Build history of the part. All positions in model axes, mm. A direction names the side the tool comes from. Give positions to 0.01 mm unless a question says otherwise; leave off trailing zeros. Loops run counter-clockwise (first coordinate to the right, second up) from the corner with the lowest first, then second, coordinate; pieces in that order, holes last. Notation, with made-up numbers: (26, 65) -> (78, 65) arc R16 cw to (78, 71) -> close; hole circle Ø3 at (26, 50.25). An arc over 180 degrees is marked (long way). Answer as a JSON object with one key per item and string values. Group by question number.
from build123d import *

# Parameters (mm, degrees)
F0_W         = 39
F0_H         = 55.5
F0_W_2       = 35
F0_H_2       = 51.5
F1_DEPTH     = 37
F3_DEPTH     = 56
F4_DEPTH     = 2
F5_R         = 2.5
F6_DEPTH     = 3
F7_W         = 6
F7_H         = 2
F8_DEPTH     = 40
F9_T1_DEPTH  = 47.5
F9_T3_DEPTH  = 31
F9_T5_DEPTH  = 43
F9_S9_W      = 4
F9_S9_H      = 4
F9_T10_DEPTH = 4
F9_S15_W     = 4
F9_S15_H     = 4
F9_T16_DEPTH = 4
F9_S21_W     = 4
F9_S21_H     = 4
F9_T22_DEPTH = 4
F9_S27_W     = 4
F9_S27_H     = 4
F9_T28_DEPTH = 4


# Not quite as in the source:
# - a fillet or chamfer that OpenCascade refuses, or shapes differently, is made with other operations: its cross-section is extruded or revolved along the edge and cut away or added


with BuildPart() as f1:
    # F0 (on Top) → F1 (new body)
    with BuildSketch(Plane.XY):
        Rectangle(F0_W, F0_H)
        Rectangle(F0_W_2, F0_H_2, mode=Mode.SUBTRACT)
    extrude(amount=F1_DEPTH)

    # F2 (on face) → F3 (cut)
    with BuildSketch(Plane(origin=(0, 27.75, 0), x_dir=(-1, 0, 0), z_dir=(0, 1, 0))):
        with BuildLine():
            Line((19.5, 37), (-19.5, 37))
            ThreePointArc((-19.5, 37), (0, 27.8760560333), (19.5, 37))
        make_face()
    extrude(amount=-F3_DEPTH, mode=Mode.SUBTRACT)

    # F0 (on Top) → F4 (join)
    with BuildSketch(Plane.XY):
        Rectangle(F0_W_2, F0_H_2)
    extrude(amount=F4_DEPTH)

    # F5 (on face) → F6 (cut)
    with BuildSketch(Plane(origin=(0, 27.75, 0), x_dir=(-1, 0, 0), z_dir=(0, 1, 0))):
        with Locations((0, 4.8760560333)):
            Circle(F5_R)
    extrude(amount=-F6_DEPTH, mode=Mode.SUBTRACT)

    # F7 (on face) → F8 (cut)
    with BuildSketch(Plane(origin=(-19.5, 0, 0), x_dir=(0, -1, 0), z_dir=(-1, 0, 0))):
        with Locations((-19.75, 31.5)):
            Rectangle(F7_W, F7_H)
        with Locations((-6.75, 31.5)):
            Rectangle(F7_W, F7_H)
        with Locations((6.25, 31.5)):
            Rectangle(F7_W, F7_H)
        with Locations((19.25, 31.5)):
            Rectangle(F7_W, F7_H)
    extrude(amount=-F8_DEPTH, mode=Mode.SUBTRACT)

    # F9: fillet of radius 4 on 8 edges, made by hand

    # F9_s2 → F9_t1 (cut)
    with BuildSketch(Plane.XZ.offset(-23.75)):
        with BuildLine():
            ThreePointArc((-15.5, 0), (-18.3284271247, 1.1715728753), (-19.5, 4))
            Line((-19.5, 4), (-19.5, 0))
            Line((-19.5, 0), (-15.5, 0))
        make_face()
        with BuildLine():
            ThreePointArc((19.5, 4), (18.3284271247, 1.1715728753), (15.5, 0))
            Line((15.5, 0), (19.5, 0))
            Line((19.5, 0), (19.5, 4))
        make_face()
    extrude(amount=F9_T1_DEPTH, mode=Mode.SUBTRACT)

    # F9_s4 → F9_t3 (cut)
    with BuildSketch(Plane.YZ.offset(-15.5)):
        with BuildLine():
            ThreePointArc((23.75, 0), (26.5784271247, 1.1715728753), (27.75, 4))
            Line((27.75, 4), (27.75, 0))
            Line((27.75, 0), (23.75, 0))
        make_face()
        with BuildLine():
            ThreePointArc((-27.75, 4), (-26.5784271247, 1.1715728753), (-23.75, 0))
            Line((-23.75, 0), (-27.75, 0))
            Line((-27.75, 0), (-27.75, 4))
        make_face()
    extrude(amount=F9_T3_DEPTH, mode=Mode.SUBTRACT)

    # F9_s6 → F9_t5 (cut)
    with BuildSketch(Plane.XY.offset(4)):
        with BuildLine():
            ThreePointArc((-15.5, -27.75), (-18.3284271247, -26.5784271247), (-19.5, -23.75))
            Line((-19.5, -23.75), (-19.5, -27.75))
            Line((-19.5, -27.75), (-15.5, -27.75))
        make_face()
        with BuildLine():
            ThreePointArc((19.5, -23.75), (18.3284271247, -26.5784271247), (15.5, -27.75))
            Line((15.5, -27.75), (19.5, -27.75))
            Line((19.5, -27.75), (19.5, -23.75))
        make_face()
        with BuildLine():
            ThreePointArc((19.5, 23.75), (18.3284271247, 26.5784271247), (15.5, 27.75))
            Line((15.5, 27.75), (19.5, 27.75))
            Line((19.5, 27.75), (19.5, 23.75))
        make_face()
        with BuildLine():
            ThreePointArc((-15.5, 27.75), (-18.3284271247, 26.5784271247), (-19.5, 23.75))
            Line((-19.5, 23.75), (-19.5, 27.75))
            Line((-19.5, 27.75), (-15.5, 27.75))
        make_face()
    extrude(amount=F9_T5_DEPTH, mode=Mode.SUBTRACT)


with BuildPart() as f9_tool8:
    # F9_s9 → F9_t10 (new body)
    with BuildSketch(Plane.XY.offset(4)):
        with Locations((-17.5, 25.75)):
            Rectangle(F9_S9_W, F9_S9_H)
    extrude(amount=-F9_T10_DEPTH)

    # F9_s11 → F9_t12 (revolve, cut)
    with BuildSketch(Plane(origin=(-15.5, 23.75, 4), x_dir=(0.7071067812, -0.7071067812, 0), z_dir=(0.7071067812, 0.7071067812, 0))):
        with BuildLine():
            ThreePointArc((0, -4), (4, 0), (0, 4))
            Line((0, 4), (0, -4))
        make_face()
    revolve(axis=Axis((-15.5, 23.75, 4), (0, 0, -1)), mode=Mode.SUBTRACT)


with BuildPart() as f1_1:
    add(f1.part)

    # F9_t7: cut F9_tool8
    add(f9_tool8.part, mode=Mode.SUBTRACT)


with BuildPart() as f9_tool14:
    # F9_s15 → F9_t16 (new body)
    with BuildSketch(Plane.XZ.offset(23.75)):
        with Locations((-17.5, 2)):
            Rectangle(F9_S15_W, F9_S15_H)
    extrude(amount=F9_T16_DEPTH)

    # F9_s17 → F9_t18 (revolve, cut)
    with BuildSketch(Plane(origin=(-15.5, -23.75, 4), x_dir=(0.7071067812, 0, 0.7071067812), z_dir=(0.7071067812, 0, -0.7071067812))):
        with BuildLine():
            ThreePointArc((0, -4), (4, 0), (0, 4))
            Line((0, 4), (0, -4))
        make_face()
    revolve(axis=Axis((-15.5, -23.75, 4), (0, -1, 0)), mode=Mode.SUBTRACT)


with BuildPart() as f1_2:
    add(f1_1.part)

    # F9_t13: cut F9_tool14
    add(f9_tool14.part, mode=Mode.SUBTRACT)


with BuildPart() as f9_tool20:
    # F9_s21 → F9_t22 (new body)
    with BuildSketch(Plane.YZ.offset(15.5)):
        with Locations((25.75, 2)):
            Rectangle(F9_S21_W, F9_S21_H)
    extrude(amount=F9_T22_DEPTH)

    # F9_s23 → F9_t24 (revolve, cut)
    with BuildSketch(Plane(origin=(15.5, 23.75, 4), x_dir=(0, -0.7071067812, 0.7071067812), z_dir=(0, 0.7071067812, 0.7071067812))):
        with BuildLine():
            ThreePointArc((0, -4), (4, 0), (0, 4))
            Line((0, 4), (0, -4))
        make_face()
    revolve(axis=Axis((15.5, 23.75, 4), (1, 0, 0)), mode=Mode.SUBTRACT)


with BuildPart() as f1_3:
    add(f1_2.part)

    # F9_t19: cut F9_tool20
    add(f9_tool20.part, mode=Mode.SUBTRACT)


with BuildPart() as f9_tool26:
    # F9_s27 → F9_t28 (new body)
    with BuildSketch(Plane.YZ.offset(15.5)):
        with Locations((-25.75, 2)):
            Rectangle(F9_S27_W, F9_S27_H)
    extrude(amount=F9_T28_DEPTH)

    # F9_s29 → F9_t30 (revolve, cut)
    with BuildSketch(Plane(origin=(15.5, -23.75, 4), x_dir=(0, 0.7071067812, 0.7071067812), z_dir=(0, 0.7071067812, -0.7071067812))):
        with BuildLine():
            ThreePointArc((0, -4), (4, 0), (0, 4))
            Line((0, 4), (0, -4))
        make_face()
    revolve(axis=Axis((15.5, -23.75, 4), (1, 0, 0)), mode=Mode.SUBTRACT)


with BuildPart() as f1_4:
    add(f1_3.part)

    # F9_t25: cut F9_tool26
    add(f9_tool26.part, mode=Mode.SUBTRACT)


solid = f1_4.part
(1) Saw through at B-B on z = 8. List the corners of the cut face in (x, y), plus the area to 3 significant figures.
(2) Probe line 1 along Y through (x, z) = (13, 15); line 2 along X through (y, z) = (-9.5, 18.5). List the from-to ranges inside material, lowest first. Write a range as [from, to].
(3) Saw through at A-A on y = -19. List the corners of the cut face in (x, z), plus the area to 3 significant figures.
(4) Pull direction Y, two halves, no side cores. Call faces 1 (the flat face through (0, -27.75, 18)), 2 (the flat face through (0, 0, 0)), 3 (the flat face through (-19, -9.25, 31)): pulls with the +Y half, pulls with the -Y half, needs draft (parallel to the pull), parting line crosses it, or undercut.
(5) 3-axis set-ups, long thin cutter, end or side, ignore diameter. For faces 4 (the cylindrical face through (0.325, 26.764, 7.355)), 5 (the cylindrical face through (18.359, 0.332, 1.203)), 6 (the flat face through (0, -25.75, 15)), 7 (the flat face through (-19, -6, 32.5)), 8 (the cylindrical face through (18.359, -26.547, 20.269)): which of +Z, -Z, +X, -X, +Y, -Y reach the whole face in a straight line?
(6) Pin check, flat tips, straight feed: pin 1 (0.6 mm diameter, centred on x = 18.5, y = 19, fed in from +Z); pin 2 (2 mm diameter, centred on x = 18, y = -18, fed in from -Z); pin 3 (0.6 mm diameter, centred on x = -18, y = 19.5, fed in from +Z); pin 4 (1.6 mm diameter, centred on x = 19, y = -18.5, fed in from +Z). Stop position of each tip, or through.
(7) Saw through at D-D on y = 13. List the corners of the cut face in (x, z), plus the area to 3 significant figures.
(8) Saw through at C-C on x = 0. List the corners of the cut face in (y, z), plus the area to 3 significant figures.
Calculated:
{
 "1": {"outline": "(-19.5, -23.75) arc R4 ccw to (-15.5, -27.75) -> (15.5, -27.75) arc R4 ccw to (19.5, -23.75) -> (19.5, 23.75) arc R4 ccw to (15.5, 27.75) -> (-15.5, 27.75) arc R4 ccw to (-19.5, 23.75) -> close; hole (-17.5, -25.75) -> (17.5, -25.75) -> (17.5, 25.75) -> (-17.5, 25.75) -> close", "area": "348 mm^2"},
 "2": {"line 1": "y = [-27.75, -25.75], [25.75, 27.75]", "line 2": "x = [-19.5, -17.5], [17.5, 19.5]"},
 "3": {"outline": "(-19.5, 4) arc R4 ccw to (-15.5, 0) -> (15.5, 0) arc R4 ccw to (19.5, 4) -> (19.5, 30.5) -> (17.5, 30.5) -> (17.5, 2) -> (-17.5, 2) -> (-17.5, 30.5) -> (-19.5, 30.5) -> close; (-19.5, 32.5) -> (-17.5, 32.5) -> (-17.5, 34.87) arc R25.4 cw to (-19.5, 37) -> close; (17.5, 32.5) -> (19.5, 32.5) -> (19.5, 37) arc R25.4 cw to (17.5, 34.87) -> close", "area": "199 mm^2"},
 "4": {"face 1": "pulls with the -Y half", "face 2": "needs draft", "face 3": "undercut"},
 "5": {"face 4": "+Y", "face 5": "-Z, +X, +Y, -Y", "face 6": "+Z", "face 7": "+X, -X", "face 8": "+Z, -Z, +X, -Y"},
 "6": {"pin 1": "stops at z = 36.2", "pin 2": "stops at z = 0.29", "pin 3": "stops at z = 35.66", "pin 4": "stops at z = 37"},
 "7": {"outline": "(-19.5, 4) arc R4 ccw to (-15.5, 0) -> (15.5, 0) arc R4 ccw to (19.5, 4) -> (19.5, 37) arc R25.4 cw to (17.5, 34.87) -> (17.5, 2) -> (-17.5, 2) -> (-17.5, 34.87) arc R25.4 cw to (-19.5, 37) -> close", "area": "207 mm^2"},
 "8": {"outline": "(-27.75, 4) arc R4 ccw to (-23.75, 0) -> (23.75, 0) arc R4 ccw to (27.41, 2.38) -> (25.75, 2.38) -> (25.75, 2) -> (-25.75, 2) -> (-25.75, 27.88) -> (-27.75, 27.88) -> close; (25.75, 7.38) -> (27.75, 7.38) -> (27.75, 27.88) -> (25.75, 27.88) -> close", "area": "198 mm^2"}
}
